from build123d import *

# Parameters (mm, degrees)
CROQUIS1_W                   = 138
CROQUIS1_H                   = 88
SALIENTE_EXTRUIR1_DEPTH      = 3
CORTAR_EXTRUIR1_REACH        = 165.698
CROQUIS2_W                   = 116
CROQUIS2_H                   = 67
TALADRO_DE_MARGEN_PARA_M31_D = 3.2


with BuildPart() as part:
    # Croquis1 → Saliente-Extruir1 (new body)
    with BuildSketch(Plane.XY):
        with Locations((69, 44)):
            Rectangle(CROQUIS1_W, CROQUIS1_H)
    extrude(amount=SALIENTE_EXTRUIR1_DEPTH)

    # Croquis2 → Cortar-Extruir1 (cut, up to next)
    with BuildSketch(Plane.XY.offset(3), mode=Mode.PRIVATE) as cortar_extruir1_sk1:
        with Locations((69, 45.5)):
            Rectangle(CROQUIS2_W, CROQUIS2_H)
    cortar_extruir1_tool1 = extrude(cortar_extruir1_sk1.sketch, amount=-CORTAR_EXTRUIR1_REACH, mode=Mode.PRIVATE) & part.part
    add(cortar_extruir1_tool1.solids().sort_by_distance((69, 45.5, 3))[0], mode=Mode.SUBTRACT)

    # Taladro de margen para M31 (through all)
    with Locations(Plane(origin=(5, 85.5, 3), x_dir=(1, 0, 0), z_dir=(0, 0, 1))):
        with Locations((0, 0), (128, 0), (128, -83), (0, -83)):
            Hole(TALADRO_DE_MARGEN_PARA_M31_D / 2)


solid = part.part
Verification items for the finished model (mm, model axes). A direction names the side the tool comes from. Coordinates: 2 decimals unless noted, no trailing zeros. Loops run counter-clockwise (first coordinate to the right, second up) from the corner with the lowest first, then second, coordinate; pieces in that order, holes last. Notation, with made-up numbers: M 32.25,61 L 43.25,61 A6 cw 43.25,71 Z; hole C -26.75,-1 d7. An arc over 180 degrees is marked long. One line per item, written item: value.
1. Mould release check, pull along Y, two halves, no side actions. Record for faces 3 (the cylindrical face through (6.27, 1.53, 1.48)), 4 (the flat face through (68, 88, 1)), 5 (the flat face through (68, 0, 1)), 6 (the flat face through (138, 43, 1)): pulls with the +Y half, pulls with the -Y half, needs draft (parallel to the pull), parting line crosses it, or undercut.
Answers follow:
face 3: undercut
face 4: pulls with the +Y half
face 5: pulls with the -Y half
face 6: needs draft
2. Section check B-B on x = 105. Record the cut outline in (y, z).
Answers follow:
outline: M 0,0 L 12,0 L 12,3 L 0,3 Z; M 79,0 L 88,0 L 88,3 L 79,3 Z
3. Section check D-D on x = 5. Record the cut outline in (y, z).
Answers follow:
outline: M 0,0 L 0.9,0 L 0.9,3 L 0,3 Z; M 4.1,0 L 83.9,0 L 83.9,3 L 4.1,3 Z; M 87.1,0 L 88,0 L 88,3 L 87.1,3 Z
4. Material ranges on line 1 along X through (y, z) = (85.5, 2); line 2 along Y through (x, z) = (133, 1); line 3 along Y through (x, z) = (40, 2.4), recorded low to high. Write a range as from..to.
Answers follow:
line 1: 0..3.4, 6.6..131.4, 134.6..138
line 2: 0..0.9, 4.1..83.9, 87.1..88
line 3: 0..12, 79..88
5. Section check A-A on y = 85.5. Record the cut outline in (x, z).
Answers follow:
outline: M 0,0 L 3.4,0 L 3.4,3 L 0,3 Z; M 6.6,0 L 131.4,0 L 131.4,3 L 6.6,3 Z; M 134.6,0 L 138,0 L 138,3 L 134.6,3 Z
6. Set-up check for faces 1 (the flat face through (68, 6, 3)), 2 (the flat face through (68, 12, 2)): record each of +Z, -Z, +X, -X, +Y, -Y from which the full face is reachable in a straight line by a thin tool's end or side.
Answers follow:
face 1: +Z, +X, -X, +Y, -Y
face 2: +Z, -Z
7. Gauge pin test, flat end, axial feed: P1, Ø1.9, axis at x = 5, y = 85.5, coming from the +Z side. Record the tip position at first contact, or that the pin passes through.
Answers follow:
P1: through
8. Section check C-C on z = 2. Record the cut outline in (x, y), plus the area to 3 significant figures.
Answers follow:
outline: M 0,0 L 138,0 L 138,88 L 0,88 Z; hole C 5,2.5 d3.2; hole C 5,85.5 d3.2; hole M 11,12 L 127,12 L 127,79 L 11,79 Z; hole C 133,2.5 d3.2; hole C 133,85.5 d3.2
area: 4,340 mm^2
